For this review, use the dimensioned drawing (mm, ordinates from the lowest corner) and the shaded views. A direction names the side the tool comes from. Round coordinates to 2 decimals unless told otherwise and drop trailing zeros. Loops run counter-clockwise (first coordinate to the right, second up) from the corner with the lowest first, then second, coordinate; pieces in that order, holes last. Notation, with made-up numbers: M 81,22 L 121,22 A15 cw 121,45 Z; hole C -2.5,77.5 d8. An arc over 180 degrees is marked long. Answer as a JSON object with one key per item and string values. Group by question number.
Item 1: Insertion check: P1, Ø2, axis at x = 46.5, y = 24.5, coming from the +Z side; P2, Ø1, axis at x = 30, y = 23.5, coming from the -Z side; P3, Ø12, axis at x = 16, z = 37, coming from the -Y side; P4, Ø10, axis at y = 18.5, z = 30.5, coming from the -X side. Each pin has a flat end and moves straight along its axis. Give the tip position at first contact, or say it passes through.
Item 2: Consider section D-D (y = 58). Give the boundary of the cut face in (x, z).
Item 3: Tool access review of the marked faces 1, 2 and 3: name each direction out of +Z, -Z, +X, -X, +Y, -Y from which nothing blocks a thin tool from reaching the whole face with its end or side.
Item 4: To check wall thickness, follow line 1 (X direction, y = 10, z = 31); line 2 (X direction, y = 5, z = 52.5). State the ranges of each line that lie inside material, in increasing order.
Item 5: Consider section A-A (z = 31.5). Give the boundary of the cut face in (x, y), and give its area (3 significant figures).
Item 6: The part is to be moulded in two halves that separate along X. For the marked faces 4 and 5, say which applies: +X half, -X half, draft (parallel to the pull), parting line (faces both ways), or undercut.
Item 7: Consider section C-C (y = 35). Give the boundary of the cut face in (x, z), and give its area (3 significant figures).
Item 8: Consider section B-B (x = 31.5). Give the boundary of the cut face in (y, z).
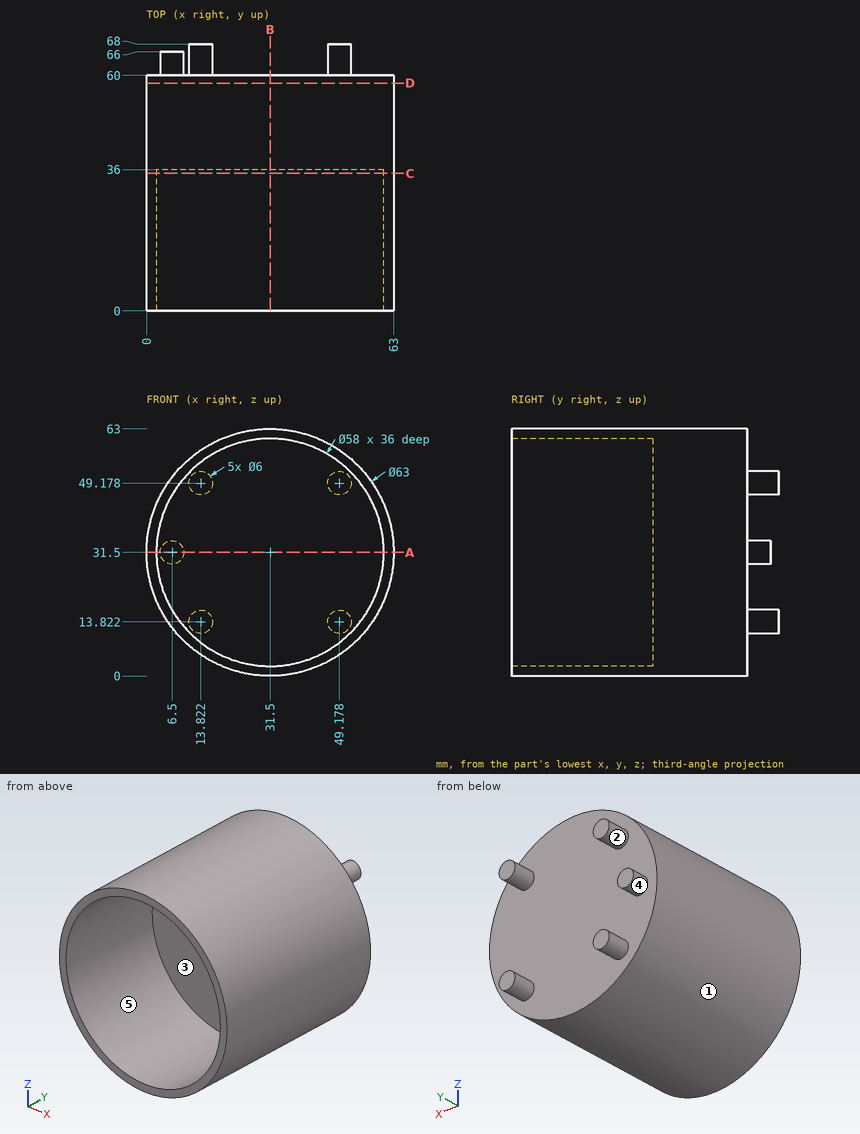
Geometry results:
{
 "1": {"P1": "stops at z = 59.72", "P2": "stops at z = 0.02", "P3": "stops at y = 36", "P4": "stops at x = 0"},
 "2": {"outline": "C 31.5,31.5 d63"},
 "3": {"face 1": "+Y, -Y", "face 2": "+Y", "face 3": "-Y"},
 "4": {"line 1": "x = 0 to 2.5, 60.5 to 63", "line 2": "x = 8.02 to 11.5, 51.5 to 54.98"},
 "5": {"outline": "M 0,0 L 2.5,0 L 2.5,36 L 60.5,36 L 60.5,0 L 63,0 L 63,60 L 9.5,60 L 9.5,66 L 3.5,66 L 3.5,60 L 0,60 Z", "area": "1,730 mm^2"},
 "6": {"face 4": "parting line", "face 5": "undercut"},
 "7": {"outline": "C 31.5,31.5 d63; hole C 31.5,31.5 d58", "area": "475 mm^2"},
 "8": {"outline": "M 0,0 L 60,0 L 60,63 L 0,63 L 0,60.5 L 36,60.5 L 36,2.5 L 0,2.5 Z"}
}
